Read the model definition and answer for the solid it produces. Units are mm, in the model's axes. A direction names the side the tool comes from. Coordinates: 2 decimals unless noted, no trailing zeros. Order: outer loops, then holes, each group sorted by start corner. A loop starts at its lowest first (then second) coordinate and runs counter-clockwise, first axis right, second up. Notation, with made-up numbers: (57, 49.25) - (112, 49.25) arc R18 ccw to (112, 58.25) - close; hole circle Ø9 at (-31, 61). An arc over 180 degrees is marked (long way). Use one line per item in the form item = value.
```python
from build123d import *

# Parameters (mm, degrees)
F0_R     = 50
F1_DEPTH = 97
F2_T     = -6
F3_R     = 2
F4_DEPTH = 40
F5_R     = 3
F6_R     = 5
F7_DEPTH = 50.001


with BuildPart() as f1:
    # F0 (on Right) → F1 (new body, symmetric)
    with BuildSketch(Plane.YZ):
        Circle(F0_R)
    extrude(amount=F1_DEPTH, both=True)

    # F2
    f2_openings = [f1.faces().sort_by_distance(p)[0] for p in [
        (97, 0, 0),
    ]]
    offset(amount=F2_T, openings=f2_openings)

    # F3 (on face) → F4 (cut)
    with BuildSketch(Plane.YZ.offset(97)):
        with Locations((-47, 0)):
            Circle(F3_R)
        with Locations((-33.234019, 33.234019)):
            Circle(F3_R)
        with Locations((0, 47)):
            Circle(F3_R)
        with Locations((33.234019, 33.234019)):
            Circle(F3_R)
        with Locations((47, 0)):
            Circle(F3_R)
        with Locations((-33.234019, -33.234019)):
            Circle(F3_R)
        with Locations((33.234019, -33.234019)):
            Circle(F3_R)
    extrude(amount=-F4_DEPTH, mode=Mode.SUBTRACT)

    # F5
    f5_edges = [f1.edges().sort_by_distance(p)[0] for p in [
        (-97, -50, 0),
    ]]
    fillet(f5_edges, radius=F5_R)

    # F6 (on Top) → F7 (cut, through all)
    with BuildSketch(Plane.XY):
        with Locations((-80, 0)):
            Circle(F6_R)
        with Locations((86, 0)):
            Circle(F6_R)
    extrude(amount=-F7_DEPTH, mode=Mode.SUBTRACT)


solid = f1.part
```
(1) Section A-A, the plane y = 0 is taken. Write down the section's boundary in (x, z), then the cut area to 3 significant figures.
Answer list:
outline = (-97, -47) arc R3 ccw to (-94, -50) - (-85, -50) - (-85, -44) - (-91, -44) - (-91, 44) - (97, 44) - (97, 45) - (57, 45) - (57, 49) - (97, 49) - (97, 50) - (-94, 50) arc R3 ccw to (-97, 47) - close; (-75, -50) - (81, -50) - (81, -44) - (-75, -44) - close; (91, -50) - (97, -50) - (97, -44) - (91, -44) - close
area = 2,570 mm2
(2) Straight lines are drawn through the part: L1, parallel to X at y = 0, z = -47; L2, parallel to X at y = 13, z = -18; L3, parallel to Z at x = 22, y = 21.5. For each, find the intervals that lie inside material, in ascending order.
Answer list:
L1 = -97 to -85, -75 to 81, 91 to 97
L2 = -97 to -91
L3 = -45.14 to -38.39, 38.39 to 45.14
(3) Section D-D, the plane x = 63.5 is taken. State how many separate pieces and enclosed holes the cut face has, then the cut area to 3 significant figures.
Answer list:
separate_pieces = 1
enclosed_holes = 8
area = 1,680 mm2
(4) Section C-C, the plane x = -48.5 is taken. Write down the section's boundary in (y, z).
Answer list:
outline = circle Ø100 at (0, 0); hole circle Ø88 at (0, 0)
(5) The mould has two halves that part along Z. Classify faces 1 (the cylindrical face through (2.84, 47.69, 15.02)), 2 (the cylindrical face through (77.28, 0.923, 45.226)), 3 (the cylindrical face through (90.619, -1.915, -46.813)): +Z half, -Z half, draft (parallel to the pull), parting line (faces both ways), or undercut.
Answer list:
face_1 = parting line
face_2 = undercut
face_3 = draft
(6) Section B-B, the plane z = 0 is taken. Write down the section's boundary in (x, y), then the cut area to 3 significant figures.
Answer list:
outline = (-97, -47) arc R3 ccw to (-94, -50) - (97, -50) - (97, -49) - (57, -49) - (57, -45) - (97, -45) - (97, -44) - (-91, -44) - (-91, 44) - (97, 44) - (97, 45) - (57, 45) - (57, 49) - (97, 49) - (97, 50) - (-94, 50) arc R3 ccw to (-97, 47) - close
area = 2,530 mm2
(7) Which of the six approach directions +Z, -Z, +X, -X, +Y, -Y give full straight-line access (tool end or side, diameter ignored) to faces 4 (the flat face through (-97, -1, 1)), 5 (the flat face through (57, 0, 47)), 6 (the cylindrical face through (-75.381, -1.915, -46.813))?
Answer list:
face_4 = +Z, -Z, -X, +Y, -Y
face_5 = +X
face_6 = -Z
(8) Given pin 1 Ø8 at (x, y) = (-29, -29.5) entering from +Z; pin 2 Ø1.2 at (y, z) = (33.5, 34) entering from +X; pin 3 Ø12 at (x, z) = (68, -9.5) entering from -Y, each flat-ended and moving along its own axis, determine where each tip first touches the part or whether it passes through.
Answer list:
pin_1 = 43.01
pin_2 = 57
pin_3 = -49.88
